from build123d import *

# Parameters (mm, degrees)
F0_W      = 20
F0_H      = 20
F3_DEPTH  = 100
F4_W      = 12.4831434727
F4_H      = 4
F5_DEPTH  = 20
F7_DEPTH  = 50
F6_R      = 2.5
F8_DEPTH  = 50
F9_W      = 4
F9_H      = 10
F10_DEPTH = 20
F11_DEPTH = 20
F12_R     = 2
F13_DEPTH = 100


with BuildPart() as f1:
    # F0 (on Front) → F1 (revolve)
    with BuildSketch(Plane.XZ):
        with Locations((10, -10)):
            Rectangle(F0_W, F0_H)
        Polygon((0, 20), (0, 0), (20, 0), (40, 0), (40, 20), align=None)
    revolve(axis=Axis((0, 0, 10), (0, 0, -1)))

    # F2 (on face) → F3 (join)
    with BuildSketch(Plane.XY.offset(20)):
        with BuildLine():
            ThreePointArc((21.6592059983, 33.6285413826), (1.9166212828, 39.9540556497), (-18.3407940017, 35.5473666449))
            Line((-18.3407940017, 35.5473666449), (-18.3407940017, -35.5473666449))
            ThreePointArc((-18.3407940017, -35.5473666449), (1.9166212828, -39.9540556497), (21.6592059983, -33.6285413826))
            Line((21.6592059983, -33.6285413826), (21.6592059983, 33.6285413826))
        make_face()
    extrude(amount=F3_DEPTH)

    # F4 (on face) → F5 (join)
    with BuildSketch(Plane.XY.offset(120)):
        with Locations((0, -10)):
            Rectangle(F4_W, F4_H)
        with Locations((0, 10)):
            Rectangle(F4_W, F4_H)
    extrude(amount=F5_DEPTH)

    # F6 (on face) → F7 (cut)
    with BuildSketch(Plane.XZ.offset(12)):
        with BuildLine():
            ThreePointArc((-6.2415717364, 130), (0, 136.2415717364), (6.2415717364, 130))
            Line((6.2415717364, 130), (6.2415717364, 140))
            Line((6.2415717364, 140), (-6.2415717364, 140))
            Line((-6.2415717364, 140), (-6.2415717364, 130))
        make_face()
    extrude(amount=-F7_DEPTH, mode=Mode.SUBTRACT)

    # F6 (on face) → F8 (cut)
    with BuildSketch(Plane.XZ.offset(12)):
        with Locations((0, 130)):
            Circle(F6_R)
    extrude(amount=-F8_DEPTH, mode=Mode.SUBTRACT)

    # F9 (on face) → F10 (join)
    with BuildSketch(Plane.YZ.offset(21.6592059983)):
        with Locations((-31.6285413826, 63.1026673317)):
            Rectangle(F9_W, F9_H)
    extrude(amount=F10_DEPTH)

    # F9 (on face) → F11 (join)
    with BuildSketch(Plane.YZ.offset(21.6592059983)):
        with Locations((31.6285413826, 63.1026673317)):
            Rectangle(F9_W, F9_H)
    extrude(amount=F11_DEPTH)

    # F12 (on face) → F13 (cut)
    with BuildSketch(Plane.XZ.offset(33.6285413826)):
        with Locations((37.3907499015, 63.1026673317)):
            Circle(F12_R)
    extrude(amount=-F13_DEPTH, mode=Mode.SUBTRACT)


solid = f1.part
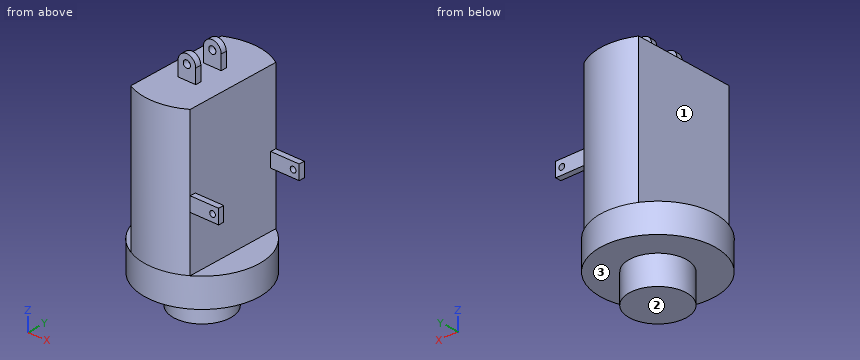
Source: CAD feature listing. Evaluate the final solid. Frame: model axes, mm. Face numbers are marked on the shaded views. A direction names the side the tool comes from. Coordinates: 2 decimals unless noted, no trailing zeros. Write each loop counter-clockwise with the first axis right and the second up, starting at its lowest first coordinate (ties: lowest second). Pieces come first, ordered by that corner, then holes. Notation, with made-up numbers: M 25,45.25 L 29,45.25 A5 ccw 29,50.25 Z; hole C 57,-3.5 d1. An arc over 180 degrees is marked long. Use a Markdown table: item, result.
1) Reachability of the marked faces 1, 2 and 3 from +Z, -Z, +X, -X, +Y, -Y: full face, straight path, thin tool, end or side. Return the list, or none.
Conclusion:
| item | result |
|---|---|
| face 1 | +Z, -X, +Y, -Y |
| face 2 | -Z, +X, -X, +Y, -Y |
| face 3 | -Z |
2) Section A-A, the plane x = 0.5. Output: boundary loops of the cut face in (y, z), then the cut area to 3 significant figures.
Conclusion:
| item | result |
|---|---|
| outline | M -40,0 L -19.99,0 L -19.99,-20 L 19.99,-20 L 19.99,0 L 40,0 L 40,120 L 12,120 L 12,127.55 L 8,127.55 L 8,120 L -8,120 L -8,127.55 L -12,127.55 L -12,120 L -40,120 Z; M -12,132.45 L -8,132.45 L -8,136.22 L -12,136.22 Z; M 8,132.45 L 12,132.45 L 12,136.22 L 8,136.22 Z |
| area | 10,500 mm^2 |
3) Ray query, L1, parallel to X at y = -10, z = 130; L2, parallel to Z at x = 0, y = 9.65; L3, parallel to Y at x = -4, z = 129.5. Return the intervals inside material, ascending.
Conclusion:
| item | result |
|---|---|
| L1 | x = -6.24 to -2.5, 2.5 to 6.24 |
| L2 | z = -20 to 127.5, 132.5 to 136.24 |
| L3 | y = -12 to -8, 8 to 12 |
4) Section C-C, the plane x = 10.5. Output: boundary loops of the cut face in (y, z).
Conclusion:
| item | result |
|---|---|
| outline | M -38.6,0 L -17.02,0 L -17.02,-20 L 17.02,-20 L 17.02,0 L 38.6,0 L 38.6,120 L -38.6,120 Z |
5) First-contact query: pin 1 Ø6 at (x, y) = (-6.5, -8.5) entering from +Z; pin 2 Ø12 at (x, y) = (-25.5, 29.5) entering from -Z; pin 3 Ø1.5 at (y, z) = (7, 10) entering from -X. Flat tips, straight axial feed; report the tip coordinate or a pass-through.
Conclusion:
| item | result |
|---|---|
| pin 1 | stops at z = 135.17 |
| pin 2 | stops at z = 0 |
| pin 3 | stops at x = -39.51 |
6) Section D-D, the plane z = 14.5. Output: boundary loops of the cut face in (x, y).
Conclusion:
| item | result |
|---|---|
| outline | C 0,0 d80 |
7) Section B-B, the plane y = 0. Output: boundary loops of the cut face in (x, z), then the cut area to 3 significant figures.
Conclusion:
| item | result |
|---|---|
| outline | M -40,0 L -20,0 L -20,-20 L 20,-20 L 20,0 L 40,0 L 40,20 L 21.66,20 L 21.66,120 L -18.34,120 L -18.34,20 L -40,20 Z |
| area | 6,400 mm^2 |
